Source: CAD feature listing. Evaluate the final solid. Frame: model axes, mm. Face numbers are marked on the shaded views. A direction names the side the tool comes from. Give positions to 0.01 mm unless a question says otherwise; leave off trailing zeros. Loops run counter-clockwise (first coordinate to the right, second up) from the corner with the lowest first, then second, coordinate; pieces in that order, holes last. Notation, with made-up numbers: (79.25, 8) -> (85.25, 8) arc R32 cw to (85.25, 36) -> close; hole circle Ø7 at (3.25, 64). An arc over 180 degrees is marked (long way). Put each result on its own line as item: value.
```python
from build123d import *

# Parameters (mm, degrees)
SKETCH1_W           = 119.38
SKETCH1_H           = 92.71
BOSS_EXTRUDE1_DEPTH = 7.62
FILLET1_R           = 2.54
SKETCH3_R           = 2.413
CUT_EXTRUDE1_DEPTH  = 8.128
SKETCH4_W           = 6.35
SKETCH4_H           = 6.35
CUT_EXTRUDE2_DEPTH  = 7.62
SKETCH5_R           = 2.54
CUT_EXTRUDE3_DEPTH  = 2.54
SKETCH6_W           = 109.728
SKETCH6_H           = 83.058
SKETCH6_W_2         = 104.648
SKETCH6_H_2         = 77.978
BOSS_EXTRUDE2_DEPTH = 2.54
SKETCH8_R           = 2.286
CUT_EXTRUDE4_DEPTH  = 8.62
SKETCH9_R           = 2.286
CUT_EXTRUDE5_DEPTH  = 8.6200001
SKETCH11_R          = 2.286
CUT_EXTRUDE6_DEPTH  = 8.6200001
SKETCH12_R          = 2.286
CUT_EXTRUDE7_DEPTH  = 8.6200001


with BuildPart() as part:
    # Sketch1 → Boss-Extrude1 (new body)
    with BuildSketch(Plane(origin=(0, 0, 0), x_dir=(1, 0, 0), z_dir=(0, 1, 0))):
        Rectangle(SKETCH1_W, SKETCH1_H)
    extrude(amount=BOSS_EXTRUDE1_DEPTH)

    # Fillet1
    fillet1_edges = [part.edges().sort_by_distance(p)[0] for p in [
        (-59.69, 7.62, 0),
        (0, 7.62, 46.355),
        (59.69, 7.62, 0),
        (0, 7.62, -46.355),
        (59.69, 3.81, 46.355),
        (-59.69, 3.81, 46.355),
        (-59.69, 3.81, -46.355),
        (59.69, 3.81, -46.355),
    ]]
    fillet(fillet1_edges, radius=FILLET1_R)

    # Sketch3 → Cut-Extrude1 (cut)
    with BuildSketch(Plane.XZ):
        with Locations((6.008676456, 29.518648142)):
            Circle(SKETCH3_R)
    extrude(amount=-CUT_EXTRUDE1_DEPTH, mode=Mode.SUBTRACT)

    # Sketch4 → Cut-Extrude2 (cut)
    with BuildSketch(Plane.XZ):
        with Locations((24.193347407, 29.518339929)):
            Rectangle(SKETCH4_W, SKETCH4_H)
    extrude(amount=-CUT_EXTRUDE2_DEPTH, mode=Mode.SUBTRACT)

    # Sketch5 → Cut-Extrude3 (cut)
    with BuildSketch(Plane(origin=(0, 7.62, 0), x_dir=(1, 0, 0), z_dir=(0, 1, 0))):
        with Locations((-57.15, -43.815)):
            Circle(SKETCH5_R)
    extrude(amount=-CUT_EXTRUDE3_DEPTH, mode=Mode.SUBTRACT)

    # Sketch6 → Boss-Extrude2 (add)
    with BuildSketch(Plane(origin=(0, 0, 0), x_dir=(-1, 0, 0), z_dir=(0, -1, 0))):
        Rectangle(SKETCH6_W, SKETCH6_H)
        Rectangle(SKETCH6_W_2, SKETCH6_H_2, mode=Mode.SUBTRACT)
    extrude(amount=BOSS_EXTRUDE2_DEPTH)

    # Sketch8 → Cut-Extrude4 (cut, through all)
    with BuildSketch(Plane.XZ):
        with Locations((56.896, 43.561)):
            Circle(SKETCH8_R)
    extrude(amount=-CUT_EXTRUDE4_DEPTH, mode=Mode.SUBTRACT)

    # Sketch9 → Cut-Extrude5 (cut, through all)
    with BuildSketch(Plane(origin=(0, 0, 0), x_dir=(-1, 0, 0), z_dir=(0, -1, 0))):
        with Locations((-56.896, 43.561)):
            Circle(SKETCH9_R)
    extrude(amount=-CUT_EXTRUDE5_DEPTH, mode=Mode.SUBTRACT)

    # Sketch11 → Cut-Extrude6 (cut, through all)
    with BuildSketch(Plane.XZ):
        with Locations((-56.896, -43.561)):
            Circle(SKETCH11_R)
    extrude(amount=-CUT_EXTRUDE6_DEPTH, mode=Mode.SUBTRACT)

    # Sketch12 → Cut-Extrude7 (cut, through all)
    with BuildSketch(Plane.XZ):
        with Locations((-56.896, 43.561)):
            Circle(SKETCH12_R)
    extrude(amount=-CUT_EXTRUDE7_DEPTH, mode=Mode.SUBTRACT)


solid = part.part
```
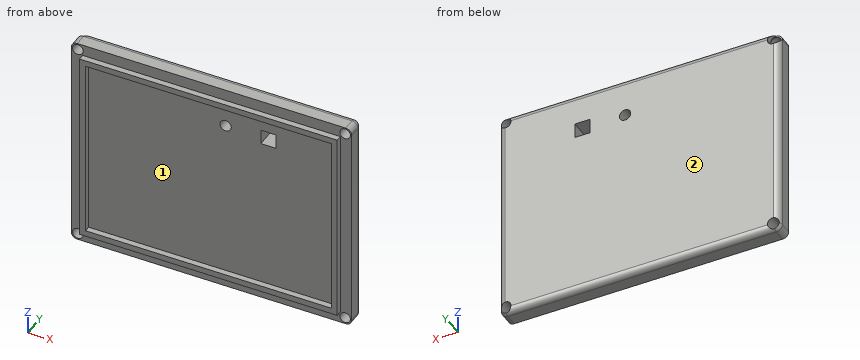
(1) Section C-C on z = 11. Return loops of the section in (x, y), then the cut area to 3 significant figures.
Calculated:
outline: (-59.69, 0) -> (-54.86, 0) -> (-54.86, -2.54) -> (-52.32, -2.54) -> (-52.32, 0) -> (52.32, 0) -> (52.32, -2.54) -> (54.86, -2.54) -> (54.86, 0) -> (59.69, 0) -> (59.69, 5.08) arc R2.54 ccw to (57.15, 7.62) -> (-57.15, 7.62) arc R2.54 ccw to (-59.69, 5.08) -> close
area: 920 mm²
(2) Section B-B on x = -6. Return loops of the section in (y, z) (3 decimals), then the cut area to 3 significant figures.
Calculated:
outline: (-2.54, -41.529) -> (0, -41.529) -> (0, -46.355) -> (5.08, -46.355) arc R2.54 ccw to (7.62, -43.815) -> (7.62, 43.815) arc R2.54 ccw to (5.08, 46.355) -> (0, 46.355) -> (0, 41.529) -> (-2.54, 41.529) -> (-2.54, 38.989) -> (0, 38.989) -> (0, -38.989) -> (-2.54, -38.989) -> close
area: 717 mm²
(3) Line query: probe 1 along X at (y, z) = (7, 30); probe 2 along X at (y, z) = (2, 27); probe 3 along X at (y, z) = (1, 42). Output: solid intervals per line, ascending. Write a range as from..to.
Calculated:
probe 1: x = -58.81..3.64, 8.37..21.02, 27.37..58.81
probe 2: x = -59.69..21.02, 27.37..59.69
probe 3: x = -59.69..-58.57, -55.23..55.23, 58.57..59.69
(4) Reachability of the marked faces 1 and 2 from +Z, -Z, +X, -X, +Y, -Y: full face, straight path, thin tool, end or side. Return the list, or none.
Calculated:
face 1: -Y
face 2: +Z, -Z, +X, -X, +Y
(5) First-contact query: P1, Ø1.3, axis at x = -9.5, y = -2, coming from the +Z side; P2, Ø2, axis at x = 27, y = -1.5, coming from the -Z side; P3, Ø5, axis at x = -38.5, z = 4, coming from the -Y side. Flat tips, straight axial feed; report the tip coordinate or a pass-through.
Calculated:
P1: stops at z = 41.53
P2: stops at z = -41.53
P3: stops at y = 0
(6) Section A-A on y = -1.25. Return loops of the section in (x, z).
Calculated:
outline: (-54.86, -41.53) -> (54.86, -41.53) -> (54.86, 41.53) -> (-54.86, 41.53) -> close; hole (-52.32, -38.99) -> (52.32, -38.99) -> (52.32, 38.99) -> (-52.32, 38.99) -> close
